Could you check a few things on this model? Use its own coordinates, in mm. A direction names the side the tool comes from. Round coordinates to 2 decimals unless told otherwise and drop trailing zeros. Loops run counter-clockwise (first coordinate to the right, second up) from the corner with the lowest first, then second, coordinate; pieces in that order, holes last.
from build123d import *

# Parameters (mm, degrees)
SKETCH1_R           = 2.65
BOSS_EXTRUDE1_DEPTH = 3
SKETCH2_R           = 1.475
BOSS_EXTRUDE2_DEPTH = 10
FILLET1_R           = 0.25
CUT_EXTRUDE1_DEPTH  = 2


with BuildPart() as part:
    # Sketch1 → Boss-Extrude1 (new body)
    with BuildSketch(Plane(origin=(0, 0, 0), x_dir=(1, 0, 0), z_dir=(0, 1, 0))):
        with Locations(Location((0, 0, 0), (0, 0, 270))):
            Circle(SKETCH1_R)
    extrude(amount=BOSS_EXTRUDE1_DEPTH)

    # Sketch2 → Boss-Extrude2 (add)
    with BuildSketch(Plane.XZ):
        with Locations(Location((0, 0, 0), (0, 0, 90))):
            Circle(SKETCH2_R)
    extrude(amount=BOSS_EXTRUDE2_DEPTH)

    # Fillet1
    fillet1_edges = [part.edges().sort_by_distance(p)[0] for p in [
        (0, 0, -2.65),
        (0, 3, -2.65),
        (0, -10, -1.475),
    ]]
    fillet(fillet1_edges, radius=FILLET1_R)

    # Sketch3 → Cut-Extrude1 (cut)
    with BuildSketch(Plane(origin=(0, 3, 0), x_dir=(1, 0, 0), z_dir=(0, 1, 0))):
        Polygon((1.732050808, 0), (0.866025404, 1.5), (-0.866025404, 1.5), (-1.732050808, 0), (-0.866025404, -1.5), (0.866025404, -1.5), align=None)
    extrude(amount=-CUT_EXTRUDE1_DEPTH, mode=Mode.SUBTRACT)


solid = part.part
Item 1: For faces 4 (the flat face through (0, 3, 2)), 5 (the flat face through (0, 1, 0)), 6 (the cylindrical face through (1.44, -4.81, -0.32)), which set-ups out of +Z, -Z, +X, -X, +Y, -Y let a thin tool reach every point of the face, with its end or its side?
Results list:
face 4: +Z, -Z, +X, -X, +Y
face 5: +Y
face 6: -Y
Item 2: If I drill on line 1 along Z through (x, y) = (-0.1, 2); line 2 along X through (y, z) = (-6.5, 0.1); line 3 along Y through (x, z) = (0.8, 0.15), over which ranges is the centre line in solid material (lowest first)?
Results list:
line 1: z = -2.65 to -1.5, 1.5 to 2.65
line 2: x = -1.47 to 1.47
line 3: y = -10 to 1
Item 3: If we section it at B-B, the plane y = -3: Please give me the cut outline in (x, z) (3 decimals), then the cut area to 3 significant figures.
Results list:
outline: circle Ø2.95 at (0, 0)
area: 6.83 mm2
Item 4: If we section it at A-A, the plane x = 0: Please give me the cut outline in (y, z) (3 decimals), then the cut area to 3 significant figures.
Results list:
outline: (-10, -1.225) arc R0.25 ccw to (-9.75, -1.475) - (0, -1.475) - (0, -2.4) arc R0.25 ccw to (0.25, -2.65) - (2.75, -2.65) arc R0.25 ccw to (3, -2.4) - (3, -1.5) - (1, -1.5) - (1, 1.5) - (3, 1.5) - (3, 2.4) arc R0.25 ccw to (2.75, 2.65) - (0.25, 2.65) arc R0.25 ccw to (0, 2.4) - (0, 1.475) - (-9.75, 1.475) arc R0.25 ccw to (-10, 1.225) - close
area: 39.3 mm2
Item 5: We'd pull the mould along Z, two halves only. Please class faces 1 (the flat face through (-2, 0, 0)), 2 (the flat face through (1.293, 2.014, 0.76)), 3 (the cylindrical face through (-1.612, 1.482, -2.103)): released by +Z, released by -Z, zero draft, split by the parting line, or undercut.
Results list:
face 1: zero draft
face 2: undercut
face 3: split by the parting line
Item 6: Will these pins go through, and if not, where does the flat tip stop? pin 1 (2 mm diameter, centred on y = -4.5, z = 1, fed in from +X) (3 decimals); pin 2 (0.5 mm diameter, centred on x = 0.5, y = 2, fed in from +Z); pin 3 (1.5 mm diameter, centred on x = 1, z = -0.5, fed in from +Y); pin 4 (1 mm diameter, centred on x = -1.5, z = -1.5, fed in from -Y).
Results list:
pin 1: stops at x = 1.475
pin 2: stops at z = 2.64
pin 3: stops at y = 3
pin 4: stops at y = 0
